Verification items for the finished model (mm, model axes). A direction names the side the tool comes from. Give positions to 0.01 mm unless a question says otherwise; leave off trailing zeros. Put each result on its own line as item: value. Start each with the question number.
from build123d import *

# Parameters (mm, degrees)
SKETCH_1_W             = 23.5
SKETCH_1_H             = 12
EXTRUDE_1_DEPTH        = 409.5
HOLE_WIZARD_M6_1_D     = 5
HOLE_WIZARD_M6_1_DEPTH = 15
HOLE_WIZARD_M6_1_TIP   = 1.502151548
HOLE_WIZARD_M6_2_D     = 5
HOLE_WIZARD_M6_2_DEPTH = 15
HOLE_WIZARD_M6_2_TIP   = 1.502151548
HOLE_WIZARD_M6_3_D     = 5
HOLE_WIZARD_M6_3_DEPTH = 15
HOLE_WIZARD_M6_3_TIP   = 1.502151548


with BuildPart() as part:
    # 草图1 → 凸台-拉伸1 (new, symmetric)
    with BuildSketch(Plane(origin=(0, 0, 0), x_dir=(0, 0, -1), z_dir=(1, 0, 0))):
        with BuildLine():
            Line((-14, 15), (-11.5, 15))
            Line((-11.5, 15), (-11.5, 13.5))
            Line((-11.5, 13.5), (-11.4, 13.5))
            ThreePointArc((-11.4, 13.5), (-11.117157288, 13.382842712), (-11, 13.1))
            Line((-11, 13.1), (-11, 12))
            Line((-11, 12), (-9.5, 12))
            Line((-9.5, 12), (-9.5, 15))
            Line((-9.5, 15), (-8, 15))
            Line((-8, 15), (-8, 12.5))
            Line((-8, 12.5), (-5, 12.5))
            Line((-5, 12.5), (-5, 15))
            Line((-5, 15), (5, 15))
            Line((5, 15), (5, 12.5))
            Line((5, 12.5), (8, 12.5))
            Line((8, 12.5), (8, 15))
            Line((8, 15), (9.5, 15))
            Line((9.5, 15), (9.5, 12))
            Line((9.5, 12), (11, 12))
            Line((11, 12), (11, 13.1))
            ThreePointArc((11, 13.1), (11.117157288, 13.382842712), (11.4, 13.5))
            Line((11.4, 13.5), (11.5, 13.5))
            Line((11.5, 13.5), (11.5, 15))
            Line((11.5, 15), (14, 15))
            ThreePointArc((14, 15), (14.707106781, 14.707106781), (15, 14))
            Line((15, 14), (15, 8))
            Line((15, 8), (12.5, 8))
            Line((12.5, 8), (12.5, 5))
            Line((12.5, 5), (15, 5))
            Line((15, 5), (15, -5))
            Line((15, -5), (12.5, -5))
            Line((12.5, -5), (12.5, -8))
            Line((12.5, -8), (15, -8))
            Line((15, -8), (15, -14))
            ThreePointArc((15, -14), (14.707106781, -14.707106781), (14, -15))
            Line((14, -15), (11.5, -15))
            Line((11.5, -15), (11.5, -13.5))
            Line((11.5, -13.5), (11.4, -13.5))
            ThreePointArc((11.4, -13.5), (11.117157288, -13.382842712), (11, -13.1))
            Line((11, -13.1), (11, -12))
            Line((11, -12), (9.5, -12))
            Line((9.5, -12), (9.5, -15))
            Line((9.5, -15), (8, -15))
            Line((8, -15), (8, -12.5))
            Line((8, -12.5), (5, -12.5))
            Line((5, -12.5), (5, -15))
            Line((5, -15), (-5, -15))
            Line((-5, -15), (-5, -12.5))
            Line((-5, -12.5), (-8, -12.5))
            Line((-8, -12.5), (-8, -15))
            Line((-8, -15), (-9.5, -15))
            Line((-9.5, -15), (-9.5, -12))
            Line((-9.5, -12), (-11, -12))
            Line((-11, -12), (-11, -13.1))
            ThreePointArc((-11, -13.1), (-11.117157288, -13.382842712), (-11.4, -13.5))
            Line((-11.4, -13.5), (-11.5, -13.5))
            Line((-11.5, -13.5), (-11.5, -15))
            Line((-11.5, -15), (-14, -15))
            ThreePointArc((-14, -15), (-14.707106781, -14.707106781), (-15, -14))
            Line((-15, -14), (-15, 14))
            ThreePointArc((-15, 14), (-14.707106781, 14.707106781), (-14, 15))
        make_face()
        with BuildLine():
            Line((12, -10.5), (12, -8.5))
            ThreePointArc((12, -8.5), (11.853553391, -8.146446609), (11.5, -8))
            Line((11.5, -8), (-11.5, -8))
            ThreePointArc((-11.5, -8), (-11.853553391, -8.146446609), (-12, -8.5))
            Line((-12, -8.5), (-12, -10.5))
            ThreePointArc((-12, -10.5), (-11.853553391, -10.853553391), (-11.5, -11))
            Line((-11.5, -11), (11.5, -11))
            ThreePointArc((11.5, -11), (11.853553391, -10.853553391), (12, -10.5))
        make_face(mode=Mode.SUBTRACT)
        with BuildLine():
            Line((-11.5, 11), (11.5, 11))
            ThreePointArc((11.5, 11), (11.853553391, 10.853553391), (12, 10.5))
            Line((12, 10.5), (12, 8.5))
            ThreePointArc((12, 8.5), (11.853553391, 8.146446609), (11.5, 8))
            Line((11.5, 8), (-11.5, 8))
            ThreePointArc((-11.5, 8), (-11.853553391, 8.146446609), (-12, 8.5))
            Line((-12, 8.5), (-12, 10.5))
            ThreePointArc((-12, 10.5), (-11.853553391, 10.853553391), (-11.5, 11))
        make_face(mode=Mode.SUBTRACT)
        Rectangle(SKETCH_1_W, SKETCH_1_H, mode=Mode.SUBTRACT)
    extrude(amount=EXTRUDE_1_DEPTH, both=True)

    # M6 螺纹孔1
    with Locations(Plane.XZ.offset(15)):
        with Locations((389.5, 0), (374.5, 0), (-192.5, 0), (-207.5, 0), (-277.5, 0), (-292.5, 0), (-374.5, 0), (-389.5, 0)):
            Hole(HOLE_WIZARD_M6_1_D / 2, depth=HOLE_WIZARD_M6_1_DEPTH)
            with Locations((0, 0, -(HOLE_WIZARD_M6_1_DEPTH + HOLE_WIZARD_M6_1_TIP / 2))):  # 118° drill point
                Cone(0, HOLE_WIZARD_M6_1_D / 2, HOLE_WIZARD_M6_1_TIP, mode=Mode.SUBTRACT)

    # M6 螺纹孔2
    with Locations(Plane(origin=(0, 0, -15), x_dir=(-1, 0, 0), z_dir=(0, 0, -1))):
        with Locations((389.5, 0), (374.5, 0), (292.5, 0), (277.5, 0), (207.5, 0), (192.5, 0)):
            Hole(HOLE_WIZARD_M6_2_D / 2, depth=HOLE_WIZARD_M6_2_DEPTH)
            with Locations((0, 0, -(HOLE_WIZARD_M6_2_DEPTH + HOLE_WIZARD_M6_2_TIP / 2))):  # 118° drill point
                Cone(0, HOLE_WIZARD_M6_2_D / 2, HOLE_WIZARD_M6_2_TIP, mode=Mode.SUBTRACT)

    # M6 螺纹孔3
    with Locations(Plane(origin=(0, 15, 0), x_dir=(-1, 0, 0), z_dir=(0, 1, 0))):
        with Locations((172.5, 0), (157.5, 0), (-374.5, 0), (-389.5, 0)):
            Hole(HOLE_WIZARD_M6_3_D / 2, depth=HOLE_WIZARD_M6_3_DEPTH)
            with Locations((0, 0, -(HOLE_WIZARD_M6_3_DEPTH + HOLE_WIZARD_M6_3_TIP / 2))):  # 118° drill point
                Cone(0, HOLE_WIZARD_M6_3_D / 2, HOLE_WIZARD_M6_3_TIP, mode=Mode.SUBTRACT)


solid = part.part
Q1. Release check for a two-part mould opening along Y. For faces 1 (the face through (6, -11, 0)), 2 (the face through (6, 11, 0)), 3 (the face through (-409.5, 7, 0)) record: pulls with the +Y half, pulls with the -Y half, needs draft (parallel to the pull), parting line crosses it, or undercut.
Q2. Scan lines: L1, parallel to Y at x = -133, z = -7.75; L2, parallel to Y at x = 190.5, z = 10; L3, parallel to Z at x = -277.5, y = -7.4. Record each from-to range of solid material in increasing order.
Q3. Go/stop test with flat-tipped pins: pin 1 (1.5 mm diameter, centred on x = -29.5, z = -6, fed in from +Y); pin 2 (0.8 mm diameter, centred on x = 37.5, z = 10.5, fed in from -Y); pin 3 (2.5 mm diameter, centred on x = 36, z = 6.5, fed in from -Y). Record where each tip stops, or that it passes through.
Q4. Set-up check for faces 4 (the face through (6, -6, 0)), 5 (the face through (6, 0, 15)): record each of +Z, -Z, +X, -X, +Y, -Y from which the full face is reachable in a straight line by a thin tool's end or side.
Q5. Cross-section at A-A, the plane x = 252.5. State how many separate pieces and enclosed holes the cut face has, then the cut area to 3 significant figures.
Ans:
1. face 1: undercut
1. face 2: undercut
1. face 3: needs draft
2. L1: y = -12.5 to -11, -8 to -6, 6 to 8, 11 to 12.5
2. L2: y = -12 to -11, -8 to -6, 6 to 8, 11 to 12
2. L3: z = -12.5 to -2.5, 2.5 to 15
3. pin 1: stops at y = 12.5
3. pin 2: stops at y = -12
3. pin 3: stops at y = -12.5
4. face 4: +X, -X
4. face 5: +Z, +X, -X, +Y, -Y
5. separate pieces: 1
5. enclosed holes: 3
5. area: 407 mm^2
